from build123d import *

# Parameters (mm, degrees)
BRIDA_BASE1_DEPTH = 25


# Sheet-metal steps are written as plain solids
with BuildPart() as part:
    # Croquis1 → Brida base1 (new body)
    with BuildSketch(Plane(origin=(0, 0, 0), x_dir=(1, 0, 0), z_dir=(0, 1, 0))):
        with BuildLine():
            ThreePointArc((9.990543733, 34.065217391), (-35.139473654, 5.046522694), (0, -35.5))
            ThreePointArc((0, -35.5), (35, -0.5), (0, 34.5))
            Line((0, 34.5), (0, 35.3))
            ThreePointArc((0, 35.3), (35.8, -0.5), (0, -36.3))
            ThreePointArc((0, -36.3), (-35.931349117, 5.160247149), (10.215682747, 34.832884262))
            Line((10.215682747, 34.832884262), (9.990543733, 34.065217391))
        make_face()
    extrude(amount=BRIDA_BASE1_DEPTH)


solid = part.part
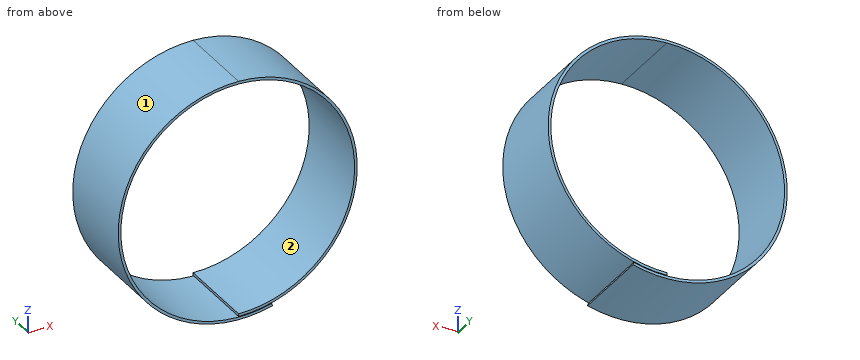
Can you work these out from the model? Positions are in its coordinate system, mm. Face numbers are marked on the shaded views. Coordinates: 2 decimals unless noted, no trailing zeros. Loops run counter-clockwise (first coordinate to the right, second up) from the corner with the lowest first, then second, coordinate; pieces in that order, holes last. Notation, with made-up numbers: M 19,88 L 51,88 A30 cw 51,124 Z; hole C -36.75,54.25 d10. An arc over 180 degrees is marked long. Return JSON: item names as keys, results as strings. Group by question number.
Item 1: Imagine slicing it at A-A (x = 28). Please give me the cut outline in (y, z), and give its area (3 significant figures).
Item 2: Imagine slicing it at C-C (y = 18.75). Please give me the cut outline in (x, z).
Item 3: Thinking about a two-plate mould opening in Z: for the marked faces 1 and 2, which applies, released by +Z, released by -Z, zero draft, split by the parting line, or undercut?
Item 4: If I drill on L1, parallel to Z at x = 1, y = 21; L2, parallel to X at y = 5.5, z = 0; L3, parallel to Z at x = 28.5, y = 5.25, over which ranges is the centre line in solid material (lowest first)? Write a range as from..to.
Item 5: Imagine slicing it at B-B (z = 22). Please give me the cut outline in (x, y).
Item 6: I'm going to push flat-ended pins straight in: pin 1 Ø1.5 at (x, y) = (27, 3.5) entering from -Z; pin 2 Ø5 at (x, y) = (-24.5, 13.5) entering from +Z; pin 3 Ø10 at (y, z) = (20, -23) entering from +X. Where does each tip first touch, or does it pass through?
Verdict:
{
 "1": {"outline": "M 0,-21.81 L 25,-21.81 L 25,-20.5 L 0,-20.5 Z; M 0,21.5 L 25,21.5 L 25,22.81 L 0,22.81 Z", "area": "65.4 mm^2"},
 "2": {"outline": "M 0,-35.3 A35.8 ccw 0,36.3 A36.3 ccw long 10.22,-34.83 L 9.99,-34.07 A35.5 cw long 0,35.5 A35 cw 0,-34.5 Z"},
 "3": {"face 1": "split by the parting line", "face 2": "undercut"},
 "4": {"L1": "z = -36.29..-35.49, -35.29..-34.49, 35.49..36.29", "L2": "x = -36.3..-35.5, 35..35.8", "L3": "z = -21.17..-19.82, 20.82..22.17"},
 "5": {"outline": "M -28.87,0 L -27.86,0 L -27.86,25 L -28.87,25 Z; M 27.62,0 L 28.62,0 L 28.62,25 L 27.62,25 Z"},
 "6": {"pin 1": "stops at z = -23.84", "pin 2": "stops at z = 28.87", "pin 3": "stops at x = 30.65"}
}
